from build123d import *

# Parameters (mm, degrees)
SKETCH1_R           = 1.5
SKETCH1_R_2         = 6
BOSS_EXTRUDE1_DEPTH = 5


with BuildPart() as part:
    # Sketch1 → Boss-Extrude1 (new body)
    with BuildSketch(Plane.XY):
        Polygon((11, 27.5), (6, 27.5), (6, 32.5), (31, 32.5), (31, 27.5), (26, 27.5), (26, 22.5), (56, 22.5), (56, 27.5), (51, 27.5), (51, 32.5), (56, 32.5), (71, 32.5), (76, 32.5), (76, 27.5), (71, 27.5), (71, 22.5), (86, 22.5), (86, -7.5), (71, -7.5), (71, -12.5), (76, -12.5), (76, -17.5), (71, -17.5), (56, -17.5), (51, -17.5), (51, -12.5), (56, -12.5), (56, -7.5), (26, -7.5), (26, -12.5), (31, -12.5), (31, -17.5), (26, -17.5), (11, -17.5), (6, -17.5), (6, -12.5), (11, -12.5), (11, -7.5), (0, -7.5), (0, 22.5), (11, 22.5), align=None)
        with Locations((32.4, 20.25)):
            Circle(SKETCH1_R, mode=Mode.SUBTRACT)
        with Locations((32.4, 2.25)):
            Circle(SKETCH1_R, mode=Mode.SUBTRACT)
        with Locations((53, 11.25)):
            Circle(SKETCH1_R_2, mode=Mode.SUBTRACT)
        with Locations((65.4, 11.25)):
            Circle(SKETCH1_R, mode=Mode.SUBTRACT)
    extrude(amount=BOSS_EXTRUDE1_DEPTH)


solid = part.part
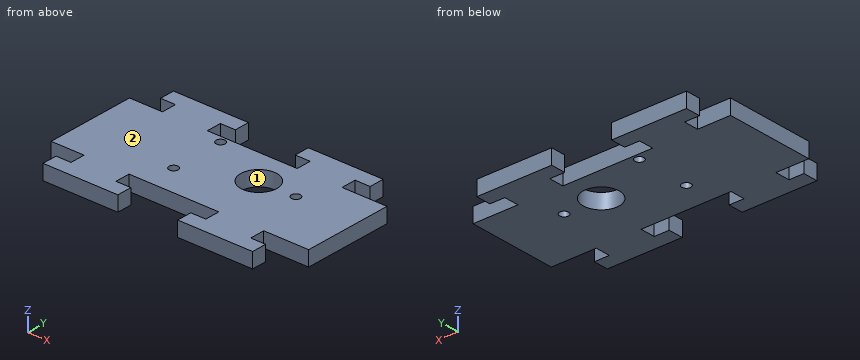
For this review, take the finished solid that the model builds, in its own axes (mm). Face numbers are marked on the shaded views. Coordinates: 2 decimals unless noted, no trailing zeros. Order: outer loops, then holes, each group sorted by start corner. A loop starts at its lowest first (then second) coordinate and runs counter-clockwise, first axis right, second up. Notation, with made-up numbers: (-33, -26.75) - (-28, -26.75) arc R9 cw to (-28, -22.75) - close; hole circle Ø10 at (82.5, 83.25). An arc over 180 degrees is marked (long way). Use one line per item in the form item = value.
Q1. Draft analysis for pull direction X (two halves, no side actions). For the marked faces 1 and 2, state which applies: +X half, -X half, draft (parallel to the pull), parting line (faces both ways), or undercut.
Checked values:
face_1 = undercut
face_2 = draft
Q2. Consider section C-C (x = 65.4). Give the boundary of the cut face in (y, z).
Checked values:
outline = (-17.5, 0) - (9.75, 0) - (9.75, 5) - (-17.5, 5) - close; (12.75, 0) - (32.5, 0) - (32.5, 5) - (12.75, 5) - close
Q3. Consider section A-A (x = 53). Give the boundary of the cut face in (y, z), then the cut area to 3 significant figures.
Checked values:
outline = (-17.5, 0) - (-12.5, 0) - (-12.5, 5) - (-17.5, 5) - close; (-7.5, 0) - (5.25, 0) - (5.25, 5) - (-7.5, 5) - close; (17.25, 0) - (22.5, 0) - (22.5, 5) - (17.25, 5) - close; (27.5, 0) - (32.5, 0) - (32.5, 5) - (27.5, 5) - close
area = 140 mm2
Q4. For P1, Ø1.5, axis at y = 26, z = 2, coming from the -X side; P2, Ø3, axis at y = -9.5, z = 1.5, coming from the +X side; P3, Ø2.5, axis at x = 79.5, z = 3.5, coming from the +Y side, all flat-tipped, find the tip position at first contact; note any pin that passes through.
Checked values:
P1 = 11
P2 = 71
P3 = 22.5
Q5. Consider section B-B (y = 11.25). Give the boundary of the cut face in (x, z), then the cut area to 3 significant figures.
Checked values:
outline = (0, 0) - (47, 0) - (47, 5) - (0, 5) - close; (59, 0) - (63.9, 0) - (63.9, 5) - (59, 5) - close; (66.9, 0) - (86, 0) - (86, 5) - (66.9, 5) - close
area = 355 mm2
Q6. Consider section D-D (y = 20.25). Give the boundary of the cut face in (x, z), then the cut area to 3 significant figures.
Checked values:
outline = (0, 0) - (30.9, 0) - (30.9, 5) - (0, 5) - close; (33.9, 0) - (86, 0) - (86, 5) - (33.9, 5) - close
area = 415 mm2
Q7. For probe 1 along Y at (x, z) = (9, 4.7); probe 2 along Y at (x, z) = (32.4, 2.5); probe 3 along X at (y, z) = (29.5, 3), list the stretches that pass through material, from the lowest coordinate up. Write a range as from..to.
Checked values:
probe_1 = -17.5..-12.5, -7.5..22.5, 27.5..32.5
probe_2 = -7.5..0.75, 3.75..18.75, 21.75..22.5
probe_3 = 6..31, 51..76
